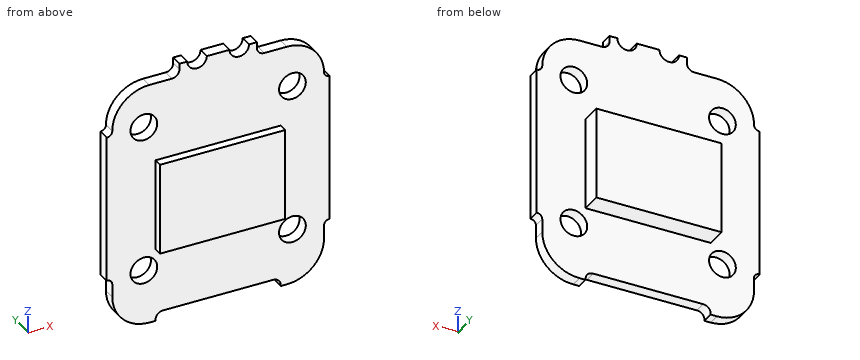
from build123d import *

# Parameters (mm, degrees)
SKETCH1_R           = 1800
BOSS_EXTRUDE1_DEPTH = 1600
SCALE1_SCALE        = 0.001
SKETCH2_W           = 16.847552216
SKETCH2_H           = 12.419052776
BOSS_EXTRUDE2_DEPTH = 2.75


with BuildPart() as part:
    # Sketch1 → Boss-Extrude1 (new body)
    with BuildSketch(Plane(origin=(0, 0, 0), x_dir=(1, 0, 0), z_dir=(0, 1, 0))):
        with BuildLine():
            Line((5206.912757967, -17500), (4155.788895153, -17500))
            ThreePointArc((4155.788895153, -17500), (2840.267529192, -16184.478634039), (1524.746163231, -17500))
            Line((1524.746163231, -17500), (-1524.746163231, -17500))
            ThreePointArc((-1524.746163231, -17500), (-2840.267529192, -16184.478634039), (-4155.788895153, -17500))
            Line((-4155.788895153, -17500), (-5206.912757967, -17500))
            Line((-5206.912757967, -17500), (-5206.912757967, -16704.41462639))
            ThreePointArc((-5206.912757967, -16704.41462639), (-5499.80597678, -15997.307845203), (-6206.912757967, -15704.41462639))
            Line((-6206.912757967, -15704.41462639), (-9252.786387289, -15704.41462639))
            ThreePointArc((-9252.786387289, -15704.41462639), (-12788.320293222, -14239.948532322), (-14252.786387289, -10704.414626389))
            Line((-14252.786387289, -10704.414626389), (-14252.786387289, -10700))
            ThreePointArc((-14252.786387289, -10700), (-14457.811640459, -10205.025253169), (-14952.786387289, -10000))
            Line((-14952.786387289, -10000), (-15000, -10000))
            Line((-15000, -10000), (-15000, 10000))
            Line((-15000, 10000), (-14952.786387289, 10000))
            ThreePointArc((-14952.786387289, 10000), (-14457.811640459, 10205.025253169), (-14252.786387289, 10700))
            Line((-14252.786387289, 10700), (-14252.786387289, 12500))
            ThreePointArc((-14252.786387289, 12500), (-12788.320293222, 16035.533905933), (-9252.786387289, 17500))
            Line((-9252.786387289, 17500), (-8419.317674219, 17500))
            Line((-8419.317674219, 17500), (-8419.317674219, 17333.689702781))
            ThreePointArc((-8419.317674219, 17333.689702781), (-8126.424455406, 16626.582921594), (-7419.317674219, 16333.689702781))
            Line((-7419.317674219, 16333.689702781), (7419.317674219, 16333.689702781))
            ThreePointArc((7419.317674219, 16333.689702781), (8126.424455406, 16626.582921594), (8419.31767422, 17333.689702781))
            Line((8419.31767422, 17333.689702781), (8419.31767422, 17500))
            Line((8419.31767422, 17500), (9252.786387289, 17500))
            ThreePointArc((9252.786387289, 17500), (12788.320293222, 16035.533905933), (14252.786387289, 12500))
            Line((14252.786387289, 12500), (14252.786387289, 10700))
            ThreePointArc((14252.786387289, 10700), (14457.811640459, 10205.02525317), (14952.786387289, 10000))
            Line((14952.786387289, 10000), (15000, 10000))
            Line((15000, 10000), (15000, -10000))
            Line((15000, -10000), (14952.786387289, -10000))
            ThreePointArc((14952.786387289, -10000), (14457.811640459, -10205.02525317), (14252.786387289, -10700))
            Line((14252.786387289, -10700), (14252.786387289, -10704.414626389))
            ThreePointArc((14252.786387289, -10704.414626389), (12788.320293222, -14239.948532322), (9252.786387289, -15704.41462639))
            Line((9252.786387289, -15704.41462639), (6206.912757967, -15704.41462639))
            ThreePointArc((6206.912757967, -15704.41462639), (5499.80597678, -15997.307845203), (5206.912757967, -16704.41462639))
            Line((5206.912757967, -16704.41462639), (5206.912757967, -17500))
        make_face()
        with Locations(Location((10000, -10000, 0), (0, 0, 270))):
            Circle(SKETCH1_R, mode=Mode.SUBTRACT)
        with Locations(Location((-10000, -10000, 0), (0, 0, 270))):
            Circle(SKETCH1_R, mode=Mode.SUBTRACT)
        with Locations(Location((-10000, 10000, 0), (0, 0, 270))):
            Circle(SKETCH1_R, mode=Mode.SUBTRACT)
        with Locations(Location((10000, 10000, 0), (0, 0, 270))):
            Circle(SKETCH1_R, mode=Mode.SUBTRACT)
    extrude(amount=BOSS_EXTRUDE1_DEPTH)


with BuildPart() as part_1:
    # Scale1: scaled about (0, 800, -308.21729277)
    add(part.part.scale(SCALE1_SCALE).moved(Location((0, 799.2, -307.909075477))))

    # Sketch2 → Boss-Extrude2 (add, symmetric)
    with BuildSketch(Plane(origin=(0, 800.8, 0), x_dir=(1, 0, 0), z_dir=(0, 1, 0))):
        with Locations((0, 309.184675859)):
            Rectangle(SKETCH2_W, SKETCH2_H)
    extrude(amount=BOSS_EXTRUDE2_DEPTH, both=True)


solid = part_1.part
The model under review builds one solid part; all positions refer to its coordinate system, in mm. Give positions to 0.01 mm unless a question says otherwise; leave off trailing zeros. Loops run counter-clockwise (first coordinate to the right, second up) from the corner with the lowest first, then second, coordinate; pieces in that order, holes last. Notation, with made-up numbers: (-33.75, 69.5) -> (2.25, 69.5) arc R17 cw to (2.25, 85.5) -> close; hole circle Ø4 at (-28, -14). An arc over 180 degrees is marked (long way). Put each result on its own line as item: value. Start each with the question number.
1. We need section C-C on y = 801.4. State the section outline as (x, z) points, then the cut area to 3 significant figures.
2. Wall thickness on probe 1 along Z at (x, y) = (-10, 800.1); probe 2 along X at (y, z) = (800.75, -318); probe 3 along Y at (x, z) = (-11, -296): over which ranges is each line inside the solid? List them lowest first.
3. We need section A-A on x = 10. State the section outline as (y, z) points.
4. Clearance check with flat-ended pins moving along their axes: P1, Ø2, axis at x = -10, z = -317.91, coming from the +Y side; P2, Ø0.8, axis at y = 802.5, z = -311.5, coming from the +X side; P3, Ø1.5, axis at x = 8, y = 802.5, coming from the +Z side; P4, Ø1.8, axis at x = 7.5, y = 800.5, coming from the +Z side. State where each tip first meets the part, or that it passes through.
5. We need section D-D on z = -299. State the section outline as (x, y) points, then the cut area to 3 significant figures.
6. We need section B-B on z = -311. State the section outline as (x, y) points, then the cut area to 3 significant figures.
Determined:
1. outline: (-8.42, -315.39) -> (8.42, -315.39) -> (8.42, -302.98) -> (-8.42, -302.98) -> close
1. area: 209 mm^2
2. probe 1: -325.35 to -319.71, -316.11 to -299.71, -296.11 to -292.26
2. probe 2: -14.61 to -11.8, -8.2 to 8.2, 11.8 to 14.61
2. probe 3: 799.2 to 800.8
3. outline: (799.2, -325.35) -> (800.8, -325.35) -> (800.8, -319.71) -> (799.2, -319.71) -> close; (799.2, -316.11) -> (800.8, -316.11) -> (800.8, -299.71) -> (799.2, -299.71) -> close; (799.2, -296.11) -> (800.8, -296.11) -> (800.8, -292.26) -> (799.2, -292.26) -> close
4. P1: through
4. P2: x = 8.42
4. P3: z = -302.98
4. P4: z = -292.2
5. outline: (-15, 799.2) -> (-11.43, 799.2) -> (-11.43, 800.8) -> (-15, 800.8) -> close; (-8.57, 799.2) -> (8.57, 799.2) -> (8.57, 800.8) -> (-8.57, 800.8) -> close; (11.43, 799.2) -> (15, 799.2) -> (15, 800.8) -> (11.43, 800.8) -> close
5. area: 38.8 mm^2
6. outline: (-15, 799.2) -> (-8.42, 799.2) -> (-8.42, 798.05) -> (8.42, 798.05) -> (8.42, 799.2) -> (15, 799.2) -> (15, 800.8) -> (8.42, 800.8) -> (8.42, 803.55) -> (-8.42, 803.55) -> (-8.42, 800.8) -> (-15, 800.8) -> close
6. area: 114 mm^2
